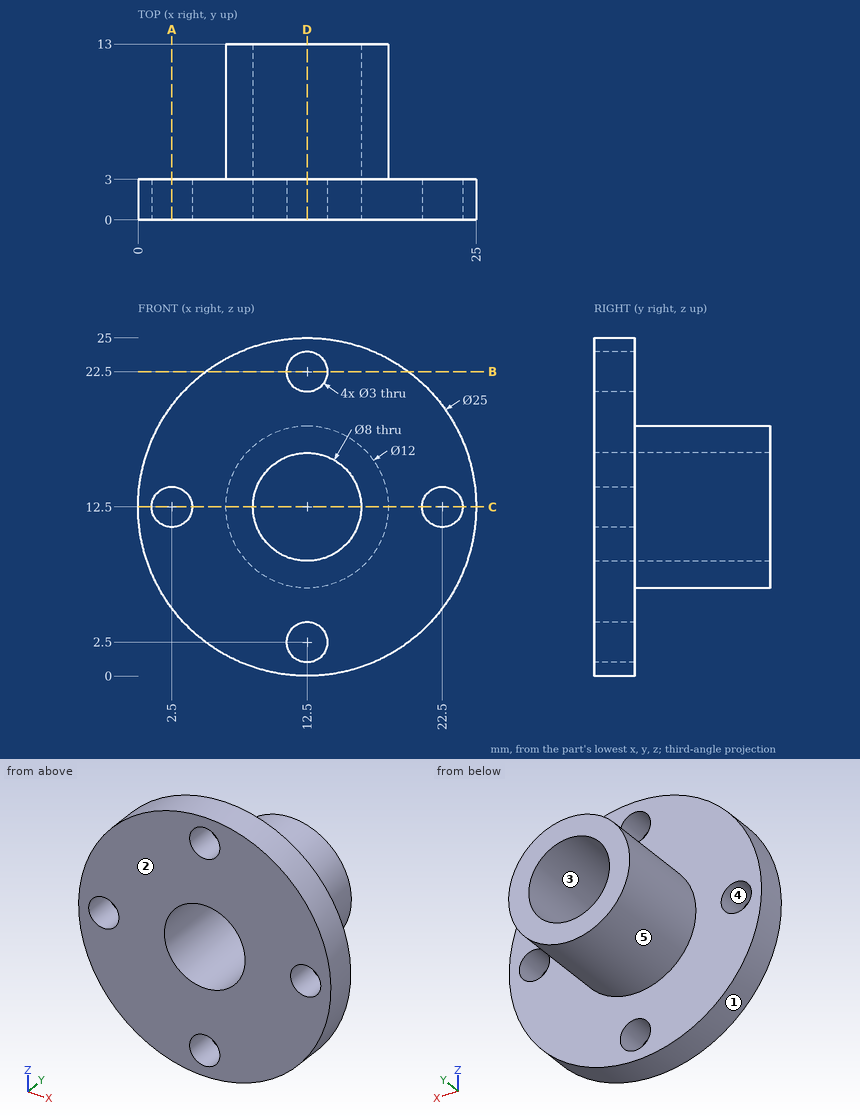
Check sheet for the drawn part. Datum: minimum x, y, z corner. Units: mm. A direction names the side the tool comes from. Give positions to 0.01 mm unless a question says otherwise; leave off trailing zeros. Loops run counter-clockwise (first coordinate to the right, second up) from the corner with the lowest first, then second, coordinate; pieces in that order, holes last. Notation, with made-up numbers: M 40,7 L 55,7 A21 ccw 55,15 Z; hole C -16,-36.75 d1. An arc over 180 degrees is marked long. Answer as CSV lines item,"result".
Item 1: Sectioned sample at A-A, the plane x = 2.5. Enter the section's corners in (y, z), then the cut area to 3 significant figures.
Reply:
outline,"M 0,5 L 3,5 L 3,11 L 0,11 Z; M 0,14 L 3,14 L 3,20 L 0,20 Z"
area,"36.0 mm^2"
Item 2: Sectioned sample at B-B, the plane z = 22.5. Enter the section's corners in (x, y), then the cut area to 3 significant figures.
Reply:
outline,"M 5,0 L 11,0 L 11,3 L 5,3 Z; M 14,0 L 20,0 L 20,3 L 14,3 Z"
area,"36.0 mm^2"
Item 3: Sectioned sample at C-C, the plane z = 12.5. Enter the section's corners in (x, y), then the cut area to 3 significant figures.
Reply:
outline,"M 0,0 L 1,0 L 1,3 L 0,3 Z; M 4,0 L 8.5,0 L 8.5,13 L 6.5,13 L 6.5,3 L 4,3 Z; M 16.5,0 L 21,0 L 21,3 L 18.5,3 L 18.5,13 L 16.5,13 Z; M 24,0 L 25,0 L 25,3 L 24,3 Z"
area,"73.0 mm^2"
Item 4: Depth check by flat-ended pin: pin 1 Ø3.5 at (x, z) = (12.5, 2.5) entering from +Y; pin 2 Ø4 at (x, y) = (6, 4.5) entering from -Z; pin 3 Ø1.5 at (x, y) = (9.5, 9) entering from +Z; pin 4 Ø2.5 at (x, z) = (22.5, 12.5) entering from -Y. Enter the tip coordinate at first touch or a pass-through.
Reply:
pin 1,"y = 3"
pin 2,"z = 1.12"
pin 3,"z = 18.06"
pin 4,"through"
Item 5: Set-up check for the marked faces 4 and 5: record each of +Z, -Z, +X, -X, +Y, -Y from which the full face is reachable in a straight line by a thin tool's end or side.
Reply:
face 4,"+Y, -Y"
face 5,"+Y"
Item 6: Scan lines: L1, parallel to X at y = 1.9, z = 12.5; L2, parallel to X at y = 5.25, z = 12.5; L3, parallel to Y at x = 10.5, z = 18.5. Record each from-to range of solid material in increasing order.
Reply:
L1,"0 to 1, 4 to 8.5, 16.5 to 21, 24 to 25"
L2,"6.5 to 8.5, 16.5 to 18.5"
L3,"0 to 3"
Item 7: Sectioned sample at D-D, the plane x = 12.5. Enter the section's corners in (y, z), then the cut area to 3 significant figures.
Reply:
outline,"M 0,0 L 3,0 L 3,1 L 0,1 Z; M 0,4 L 3,4 L 3,6.5 L 13,6.5 L 13,8.5 L 0,8.5 Z; M 0,16.5 L 13,16.5 L 13,18.5 L 3,18.5 L 3,21 L 0,21 Z; M 0,24 L 3,24 L 3,25 L 0,25 Z"
area,"73.0 mm^2"
Item 8: Draft check along Z on the marked faces 1, 2 and 3. Enter one of: pulls with the +Z half, pulls with the -Z half, needs draft (parallel to the pull), parting line crosses it, or undercut.
Reply:
face 1,"parting line crosses it"
face 2,"needs draft"
face 3,"undercut"
